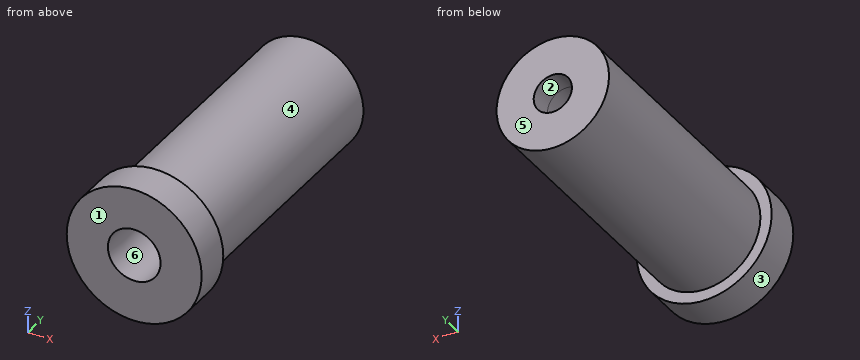
from build123d import *

# Parameters (mm, degrees)
CUT_EXTRUDE1_REACH = 43.976
SKETCH2_R          = 2.55


with BuildPart() as part:
    # Sketch1 → Revolve1 (revolve)
    with BuildSketch(Plane.XY, mode=Mode.PRIVATE) as revolve1_sk:
        Polygon((0, 0), (9, 0), (9, 5), (7.5, 5), (7.5, 40), (0, 40), align=None)
    revolve(revolve1_sk.sketch.rotate(Axis((0, 45, 0), (0, -1, 0)), 180), axis=Axis((0, 45, 0), (0, -1, 0)))

    # Sketch2 → Cut-Extrude1 (cut, up to next)
    with BuildSketch(Plane(origin=(0, 40, 0), x_dir=(1, 0, 0), z_dir=(0, 1, 0)), mode=Mode.PRIVATE) as cut_extrude1_sk1:
        with Locations(Location((0, 0, 0), (0, 0, 270))):
            Circle(SKETCH2_R)
    cut_extrude1_tool1 = extrude(cut_extrude1_sk1.sketch, amount=-CUT_EXTRUDE1_REACH, mode=Mode.PRIVATE) & part.part
    add(cut_extrude1_tool1.solids().sort_by_distance((0, 40, 0))[0], mode=Mode.SUBTRACT)

    # Cut-Sweep1: sweep along a path in Sketch5
    with BuildLine(Plane(origin=(0, 40, 0), x_dir=(1, 0, 0), z_dir=(0, 1, 0))) as cut_sweep1_path:
        CenterArc((0, 0), 2.55, 0, 360)
    # Sketch3 → Cut-Sweep1 (sweep, cut)
    with BuildSketch(Plane.XY):
        Polygon((2.55, 36.8), (3.513641914, 0), (2.55, 0), align=None)
    sweep(path=cut_sweep1_path.line, mode=Mode.SUBTRACT)


solid = part.part
Model file for the job. Use its own axes, mm. Face numbers are marked on the shaded views. A direction names the side the tool comes from. Coordinates: 2 decimals unless noted, no trailing zeros. Order: outer loops, then holes, each group sorted by start corner. A loop starts at its lowest first (then second) coordinate and runs counter-clockwise, first axis right, second up. Notation, with made-up numbers: M -2,88.5 L 5,88.5 A21 ccw 5,107.5 Z; hole C -37.75,-13 d1. An arc over 180 degrees is marked long. Return JSON: item names as keys, results as strings.
1. Pull direction Z, two halves, no side cores. Call the marked faces 1, 2 and 3: +Z half, -Z half, draft (parallel to the pull), parting line (faces both ways), or undercut.
Ans:
{"face 1": "draft", "face 2": "undercut", "face 3": "parting line"}
2. Saw through at B-B (x = 0). Give the cut face in (y, z).
Ans:
{"outline": "M 0,-9 L 5,-9 L 5,-7.5 L 40,-7.5 L 40,-2.55 L 36.8,-2.55 L 0,-3.51 Z; M 0,3.51 L 36.8,2.55 L 40,2.55 L 40,7.5 L 5,7.5 L 5,9 L 0,9 Z"}
3. Saw through at C-C (z = 6). Give the cut face in (x, y).
Ans:
{"outline": "M -6.71,0 L 6.71,0 L 6.71,5 L 4.5,5 L 4.5,40 L -4.5,40 L -4.5,5 L -6.71,5 Z"}
4. Saw through at D-D (y = 30.5). Give the cut face in (x, z).
Ans:
{"outline": "C 0,0 d15; hole C 0,0 d5.43"}
5. Saw through at A-A (z = 0). Give the cut face in (x, y).
Ans:
{"outline": "M -9,0 L -3.51,0 L -2.55,36.8 L -2.55,40 L -7.5,40 L -7.5,5 L -9,5 Z; M 2.55,36.8 L 3.51,0 L 9,0 L 9,5 L 7.5,5 L 7.5,40 L 2.55,40 Z"}
6. Drill centre lines: probe 1 along Z at (x, y) = (0, 38.95); probe 2 along Y at (x, z) = (-5, -6.5); probe 3 along X at (y, z) = (34, -0.5). Where is each one in solid material? Low to high.
Ans:
{"probe 1": "-7.5 to -2.55, 2.55 to 7.5", "probe 2": "0 to 5", "probe 3": "-7.48 to -2.58, 2.58 to 7.48"}
7. Flat gauge pins, fed straight in: pin 1 (2 mm diameter, centred on y = 10, z = 6, fed in from -X); pin 2 (8 mm diameter, centred on y = 16, z = 2, fed in from +X); pin 3 (2 mm diameter, centred on x = -1, y = 27, fed in from +Z). Where does each tip first touch, or does it go through?
Ans:
{"pin 1": "x = -5.59", "pin 2": "x = 7.5", "pin 3": "z = 7.5"}
8. Tool access for the marked faces 4, 5 and 6: list every direction of +Z, -Z, +X, -X, +Y, -Y with a clear straight run to the whole face (end or side of a thin tool).
Ans:
{"face 4": "+Y", "face 5": "+Z, -Z, +X, -X, +Y", "face 6": "-Y"}
